Input: part model. Units: mm. Frame: model coordinates. A direction names the side the tool comes from. Coordinates: 2 decimals unless noted, no trailing zeros. Loops run counter-clockwise (first coordinate to the right, second up) from the corner with the lowest first, then second, coordinate; pieces in that order, holes last.
(1) Mould query, pull axis Y, two halves, no side actions, for faces 1 (the face through (-9.609, -33.297, 1.014)), 2 (the face through (10.06, -44.357, 0.986)), 3 (the face through (13.324, -14.839, 0.986)), 4 (the face through (9.562, 9.508, 0.986)). Classes: released by +Y, released by -Y, zero draft, split by the parting line, or undercut.
(2) Line query: L1, parallel to X at y = -18, z = 1.5; L2, parallel to Y at x = 13.5, z = 1.1; L3, parallel to Y at x = -1.5, z = 1.95. Output: solid intervals per line, ascending.
(3) Section D-D, the plane y = 1. Return loops of the section in (x, z).
(4) Contact query for flat-ended pins moving along their axis: P1, Ø0.6, axis at x = 1, z = 0.5, coming from the +Y side; P2, Ø4.5, axis at x = 13.5, y = -13.5, coming from the -Z side; P3, Ø1, axis at x = 3.5, y = 6, coming from the +Z side. Output: stop coordinate, or through.
(5) Section C-C, the plane x = 0. Return loops of the section in (y, z), then the cut area to 3 significant figures.
(6) Section A-A, the plane z = 0.7. Give the number of separate pieces and of enclosed holes in the cut face, then the cut area to 3 significant figures.
(7) Section B-B, the plane y = -8. Return loops of the section in (x, z), then the cut area to 3 significant figures.
(8) Set-up query: faces 5 (the face through (6.24, -45.46, 1.01)), 6 (the face through (-6.3, -40, 1)). Return all of +Z, -Z, +X, -X, +Y, -Y with unobstructed straight access to the full face (end or side cutting, diameter ignored); none if empty.
Autodesk Inventor part; units mm, degrees
ref_plane "YZ Plane" through (0, 0, 0) normal (1, 0, 0) x (0, 1, 0)
ref_plane "XZ Plane" through (0, 0, 0) normal (0, 1, 0) x (-1, 0, 0)
ref_plane "XY Plane" through (0, 0, 0) normal (0, 0, 1) x (1, 0, 0)
sketch "スケッチ1" plane through (0, 0, 0) normal (0, 0, 1) x (1, 0, 0)
  line L0 (-13.5, 13.5) -> (13.5, 13.5) construction
  line L1 (13.5, 13.5) -> (13.5, -13.5) construction
  line L2 (13.5, -13.5) -> (-13.5, -13.5) construction
  line L3 (-13.5, -13.5) -> (-13.5, 13.5) construction
  circle A0 centre (-13.5, 13.5) radius 1.35
  circle A1 centre (13.5, 13.5) radius 1.35
  circle A2 centre (-13.5, -13.5) radius 1.35
  circle A3 centre (13.5, -13.5) radius 1.35
  circle A4 centre (0, 14.5) radius 10.5 construction
  line L4 (-6.25, -37.5) -> (6.25, -37.5) construction
  line L5 (6.25, -37.5) -> (6.25, -42.5) construction
  line L6 (6.25, -42.5) -> (-6.25, -42.5) construction
  line L7 (-6.25, -42.5) -> (-6.25, -37.5) construction
  line L8 (-16.25, -37.5) -> (16.25, -37.5) construction
  line L9 (16.25, -37.5) -> (16.25, -42.5) construction
  line L10 (16.25, -42.5) -> (-16.25, -42.5) construction
  line L11 (-16.25, -42.5) -> (-16.25, -37.5) construction
  line L12 (-6.3, -37.45) -> (6.3, -37.45) construction
  line L13 (6.3, -37.45) -> (6.3, -42.55) construction
  line L14 (6.3, -42.55) -> (-6.3, -42.55) construction
  line L15 (-6.3, -42.55) -> (-6.3, -37.45) construction
  circle A5 centre (-5.25, -37.45) radius 1.05 construction
  circle A6 centre (-11.25, -40) radius 1.55
  circle A7 centre (11.25, -40) radius 1.55
  line L16 (0, 0) -> (0, -13.5) construction
  line L17 (-6.3, -37.45) -> (-6.3, -42.55)
  line L18 (6.3, -40) -> (-6.3, -40) construction
  line L19 (0, -37.5) -> (0, -42.55) construction
  arc A8 (-4.2, -37.45) -> (-6.3, -37.45) centre (-5.25, -37.45) ccw
  arc A9 (-6.3, -42.55) -> (-4.2, -42.55) centre (-5.25, -42.55) ccw
  line L20 (-4.2, -37.45) -> (4.2, -37.45)
  line L21 (-4.2, -42.55) -> (4.2, -42.55)
  arc A10 (6.3, -37.45) -> (4.2, -37.45) centre (5.25, -37.45) ccw
  arc A11 (4.2, -42.55) -> (6.3, -42.55) centre (5.25, -42.55) ccw
  line L22 (6.3, -37.45) -> (6.3, -42.55)
  circle A12 centre (-13.5, -13.5) radius 2.75 construction
  circle A13 centre (13.5, 13.5) radius 2.75 construction
  line L23 (-16.25, -13.5) -> (-16.25, -42.5)
  line L24 (-16.25, -42.5) -> (-6.25, -45.5)
  line L25 (-6.25, -45.5) -> (6.25, -45.5)
  line L26 (6.25, -45.5) -> (16.25, -42.5)
  line L27 (16.25, -42.5) -> (16.25, 13.5)
  arc A14 (16.25, 13.5) -> (10.7575, 13.7031) centre (13.5, 13.5) ccw
  arc A15 (6.7066, 6.0513) -> (10.7575, 13.7031) centre (0, 14.5) ccw
  line L28 (6.7066, 6.0513) -> (-15.2098, -11.3461)
  arc A16 (-15.2098, -11.3461) -> (-16.25, -13.5) centre (-13.5, -13.5) ccw
  line L29 (-10.75, -14.1897) -> (-10.75, -34.5)
  line L30 (-10.75, -34.5) -> (10.75, -34.5)
  line L31 (10.75, -34.5) -> (10.75, 2.8772)
  line L32 (10.75, 2.8772) -> (-10.75, -14.1897)
  point P0 (0, 13.5)
  point P1 (13.5, 0)
  point P2 (-16.25, -40)
  dimension "d23" = 2.1
  dimension "d0" = 27
  dimension "d3" = 27
  dimension "d6" = 27
  dimension "d9" = 2.7
  dimension "d10" = 21
  dimension "d11" = 1
  dimension "d12" = 24
  dimension "d13" = 5
  dimension "d16" = 32.5
  dimension "d20" = 10
  dimension "d22" = 0.05
  dimension "d24" = 5
  dimension "d26" = 3.1
  dimension "d31" = 5.5
  dimension "d32" = 3
  dimension "d33" = 5
  dimension "d34" = 3
extrude "押し出し1" add sketch "スケッチ1" along normal blind 2 contours A16 L28 A15 A14 L27 L26 L25 L24 L23
fillet "フィレット1" radius 4 8 edges at (10.75, 2.8772, 1) (-10.75, -34.5, 1) (-10.75, -14.1897, 1) (10.75, -34.5, 1) (16.25, -42.5, 1) (-16.25, -42.5, 1) (-6.25, -45.5, 1) (6.25, -45.5, 1)
equation "\"d3\" = d0"
equation "\"d6\" = d0"
equation "\"d16\" = d0_1"
equation "\"d20\" = d3_1"
equation "\"d24\" = d17"
equation "\"d34\" = d32"
properties part number "上腕_サブフレーム_1_1" material "GFRP"
Report:
1. face 1: undercut
1. face 2: released by -Y
1. face 3: undercut
1. face 4: released by +Y
2. L1: x = -16.25 to -10.75, 10.75 to 16.25
2. L2: y = -43.32 to -14.85, -12.15 to 12.15, 14.85 to 16.25
2. L3: y = -45.5 to -42.55, -37.45 to -34.5, -6.85 to -0.46
3. outline: (0.34, 0) - (16.25, 0) - (16.25, 2) - (0.34, 2) - close
4. P1: stops at y = 1.76
4. P2: stops at z = 0
4. P3: passes through
5. outline: (-45.5, 0) - (-42.55, 0) - (-42.55, 2) - (-45.5, 2) - close; (-37.45, 0) - (-34.5, 0) - (-34.5, 2) - (-37.45, 2) - close; (-5.66, 0) - (0.73, 0) - (0.73, 2) - (-5.66, 2) - close
5. area: 24.6 mm2
6. separate pieces: 1
6. enclosed holes: 7
6. area: 795 mm2
7. outline: (-10.99, 0) - (-2.95, 0) - (-2.95, 2) - (-10.99, 2) - close; (10.75, 0) - (16.25, 0) - (16.25, 2) - (10.75, 2) - close
7. area: 27.1 mm2
8. face 5: +Z, -Z, +X, -Y
8. face 6: +Z, -Z
